from build123d import *
from build123d import SkipClean  # not in build123d's __all__

# Parameters (mm, degrees)
F1_DEPTH = 1.5
F2_W     = 2
F2_H     = 23.5
F3_DEPTH = 8
F4_W     = 1
F4_H     = 23.5
F5_DEPTH = 5
F7_DEPTH = 1
F9_DEPTH = 2.5


# Not quite as in the source:
# - a feature names something its author has since deleted; it is built from what else it names


with BuildPart() as f1:
    # F0 (on Top) → F1 (new body)
    with BuildSketch(Plane.XY):
        with BuildLine():
            ThreePointArc((0, 9.25), (-3.25, 12.5), (0, 15.75))
            Line((0, 15.75), (0, 24.5))
            Line((0, 24.5), (-11.7, 24.5))
            Line((-11.7, 24.5), (-11.7, 0))
            Line((-11.7, 0), (0, 0))
            Line((0, 0), (0, 9.25))
        make_face()
    extrude(amount=F1_DEPTH)

    # F2 (on face) → F3 (join)
    with BuildSketch(Plane.XY.offset(1.5)):
        with Locations((-9.5, 11.75)):
            Rectangle(F2_W, F2_H)
    extrude(amount=F3_DEPTH)

    # F4 (on face) → F5 (join)
    with BuildSketch(Plane.XY.offset(9.5)):
        with Locations((-10, 11.75)):
            Rectangle(F4_W, F4_H)
    extrude(amount=F5_DEPTH)

    # F6 (on face) → F7 (join)
    with BuildSketch(Plane(origin=(0, 23.5, 0), x_dir=(-1, 0, 0), z_dir=(0, 1, 0))):
        Polygon((9.5, 9.5), (9.5, 14.5), (3.5, 14.5), (3.5, 10), (8.5, 6), (8.5, 9.5), align=None)
    extrude(amount=-F7_DEPTH)

    # F8 (on face) → F9 (join)
    with BuildSketch(Plane.XZ.offset(-22.5)):
        Polygon((-8.5, 14.5), (-9.5, 14.5), (-9.5, 12.5), (-8.5, 13.5), align=None)
    extrude(amount=F9_DEPTH)

    # F10: F1 across plane


with BuildPart() as f1_1:
    add(f1.part, clean=False)
    add(f1.part.mirror(Plane.XZ), clean=False)

    # F11: F1 across plane


with BuildPart() as f1_2:
    add(f1_1.part, clean=False)
    with SkipClean():  # cleaning this boolean's faces spoils the solid; the shape is the same uncleaned
        add(f1_1.part.mirror(Plane.YZ), clean=False)


solid = f1_2.part
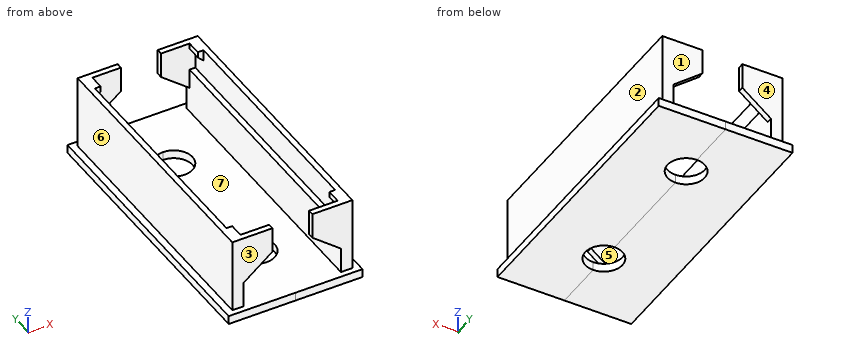
Model file for the job. Use its own axes, mm. Face numbers are marked on the shaded views. A direction names the side the tool comes from. Coordinates: 2 decimals unless noted, no trailing zeros. Loops run counter-clockwise (first coordinate to the right, second up) from the corner with the lowest first, then second, coordinate; pieces in that order, holes last. Notation, with made-up numbers: (34.5, 52.5) -> (83.5, 52.5) arc R7 ccw to (83.5, 56.5) -> close; hole circle Ø3 at (-1.75, 20.25). An arc over 180 degrees is marked (long way). Use one line per item in the form item = value. Start each with the question number.
(1) Cut at A-A on z = 13. Give the cut face in (x, y).
(2) Probe probe 1 along Y at (x, z) = (-6, 10.75); probe 2 along X at (y, z) = (0, 5.5); probe 3 along X at (y, z) = (-11.5, 9.75). List the from-to ranges inside material, lowest first. Write a range as from..to.
(3) Pull direction X, two halves, no side cores. Call the marked faces 4, 5, 6 and 7: pulls with the +X half, pulls with the -X half, needs draft (parallel to the pull), parting line crosses it, or undercut.
(4) Cut at C-C on y = -19. Give the cut face in (x, z).
(5) Flat gauge pins, fed straight in: pin 1 (3 mm diameter, centred on x = 6, z = 9, fed in from +Y); pin 2 (1.1 mm diameter, centred on y = 21.5, z = 14, fed in from +X); pin 3 (1 mm diameter, centred on x = -1, y = 5, fed in from +Z). Where does each tip first touch, or does it go through?
(6) Tool access for the marked faces 1, 2 and 3: list every direction of +Z, -Z, +X, -X, +Y, -Y with a clear straight run to the whole face (end or side of a thin tool).
(7) Cut at B-B on y = -12.5. Give the cut face in (x, z).
(8) Cut at D-D on y = 15. Give the cut face in (x, z).
Values:
q1.outline = (-10.5, -23.5) -> (-3.5, -23.5) -> (-3.5, -22.5) -> (-9, -22.5) -> (-9, -20) -> (-9.5, -20) -> (-9.5, 20) -> (-9, 20) -> (-9, 22.5) -> (-3.5, 22.5) -> (-3.5, 23.5) -> (-10.5, 23.5) -> close; (3.5, -23.5) -> (10.5, -23.5) -> (10.5, 23.5) -> (3.5, 23.5) -> (3.5, 22.5) -> (9, 22.5) -> (9, 20) -> (9.5, 20) -> (9.5, -20) -> (9, -20) -> (9, -22.5) -> (3.5, -22.5) -> close
q2.probe_1 = -23.5..-22.5, 22.5..23.5
q2.probe_2 = -10.5..-8.5, 8.5..10.5
q2.probe_3 = -10.5..-9.5, 9.5..10.5
q3.face_4 = needs draft
q3.face_5 = undercut
q3.face_6 = pulls with the -X half
q3.face_7 = undercut
q4.outline = (-11.7, 0) -> (11.7, 0) -> (11.7, 1.5) -> (10.5, 1.5) -> (10.5, 14.5) -> (9.5, 14.5) -> (9.5, 9.5) -> (8.5, 9.5) -> (8.5, 1.5) -> (-8.5, 1.5) -> (-8.5, 9.5) -> (-9.5, 9.5) -> (-9.5, 14.5) -> (-10.5, 14.5) -> (-10.5, 1.5) -> (-11.7, 1.5) -> close
q5.pin_1 = 23.5
q5.pin_2 = 10.5
q5.pin_3 = 1.5
q6.face_1 = +Z, +X, -X, +Y
q6.face_2 = +Z, +X, +Y, -Y
q6.face_3 = +Z, +X, -X, -Y
q7.outline = (-11.7, 0) -> (-3.25, 0) -> (-3.25, 1.5) -> (-8.5, 1.5) -> (-8.5, 9.5) -> (-9.5, 9.5) -> (-9.5, 14.5) -> (-10.5, 14.5) -> (-10.5, 1.5) -> (-11.7, 1.5) -> close; (3.25, 0) -> (11.7, 0) -> (11.7, 1.5) -> (10.5, 1.5) -> (10.5, 14.5) -> (9.5, 14.5) -> (9.5, 9.5) -> (8.5, 9.5) -> (8.5, 1.5) -> (3.25, 1.5) -> close
q8.outline = (-11.7, 0) -> (-2.08, 0) -> (-2.08, 1.5) -> (-8.5, 1.5) -> (-8.5, 9.5) -> (-9.5, 9.5) -> (-9.5, 14.5) -> (-10.5, 14.5) -> (-10.5, 1.5) -> (-11.7, 1.5) -> close; (2.08, 0) -> (11.7, 0) -> (11.7, 1.5) -> (10.5, 1.5) -> (10.5, 14.5) -> (9.5, 14.5) -> (9.5, 9.5) -> (8.5, 9.5) -> (8.5, 1.5) -> (2.08, 1.5) -> close
